from build123d import *

# Parameters (mm, degrees)
SKETCH044_R       = 1.6
PAD025_DEPTH      = 9
FILLET013_R       = 1
SKETCH075_W       = 8
SKETCH075_H       = 3
POCKET_DEPTH      = 37.001
POCKET_DEPTH_BACK = -17.001
CHAMFER_SIZE      = 0.4


with BuildPart() as part:
    # Sketch044 → Pad025 (new body)
    with BuildSketch(Plane.YZ):
        Polygon((-10, 17), (13, 17), (13, -37), (-10, -37), (-10, -30), (10, -30), (10, 10), (-10, 10), align=None)
        with Locations((-5, 14.5)):
            Circle(SKETCH044_R, mode=Mode.SUBTRACT)
        with Locations((5, 14.5)):
            Circle(SKETCH044_R, mode=Mode.SUBTRACT)
        with Locations((-5, -34.5)):
            Circle(SKETCH044_R, mode=Mode.SUBTRACT)
        with Locations((5, -34.5)):
            Circle(SKETCH044_R, mode=Mode.SUBTRACT)
    extrude(amount=-PAD025_DEPTH)

    # Fillet013
    fillet013_edges = [part.edges().sort_by_distance(p)[0] for p in [
        (-4.5, -10, 17),
        (-4.5, -10, 10),
        (-4.5, -10, -30),
        (-4.5, -10, -37),
        (-4.5, 13, -37),
        (-4.5, 13, 17),
    ]]
    fillet(fillet013_edges, radius=FILLET013_R)

    # Sketch075 (on XY_Plane042 of Origin045) → Pocket (cut, two sides)
    with BuildSketch(Plane.XY) as pocket_sk:
        Rectangle(SKETCH075_W, SKETCH075_H)
    extrude(amount=-POCKET_DEPTH, mode=Mode.SUBTRACT)
    extrude(pocket_sk.sketch, amount=-POCKET_DEPTH_BACK, mode=Mode.SUBTRACT)

    # Chamfer
    chamfer_edges = [part.edges().sort_by_distance(p)[0] for p in [
        (0, 6.75, 17),
        (0, 12.707107, 16.707107),
        (0, 13, -10),
        (0, 12.707107, -36.707107),
        (0, 6.75, -37),
        (0, 1.5, -33.5),
        (0, 5.75, -30),
        (0, 10, -10),
        (0, 5.75, 10),
        (0, 1.5, 13.5),
        (0, 3.4, -34.5),
        (0, 3.4, 14.5),
        (0, -5.25, 17),
        (0, -1.5, 13.5),
        (0, -5.25, 10),
        (0, -9.707107, 10.292893),
        (0, -10, 13.5),
        (0, -9.707107, 16.707107),
        (0, -6.6, 14.5),
        (0, -1.5, -33.5),
        (0, -5.25, -37),
        (0, -9.707107, -36.707107),
        (0, -10, -33.5),
        (0, -9.707107, -30.292893),
        (0, -5.25, -30),
        (0, -6.6, -34.5),
        (-9, 1.5, 17),
        (-9, -9.707107, 16.707107),
        (-9, 12.707107, 16.707107),
        (-9, -10, 13.5),
        (-9, 13, -10),
        (-9, -9.707107, 10.292893),
        (-9, 12.707107, -36.707107),
        (-9, 0.5, 10),
        (-9, 1.5, -37),
        (-9, 10, -10),
        (-9, -9.707107, -36.707107),
        (-9, 0.5, -30),
        (-9, -10, -33.5),
        (-9, -9.707107, -30.292893),
        (-9, -6.6, 14.5),
        (-9, 3.4, 14.5),
        (-9, -6.6, -34.5),
        (-9, 3.4, -34.5),
    ]]
    chamfer(chamfer_edges, length=CHAMFER_SIZE)


solid = part.part
Geometry: final body of the model. Coordinates: model frame, mm. A direction names the side the tool comes from. Give positions to 0.01 mm unless a question says otherwise; leave off trailing zeros. Order: outer loops, then holes, each group sorted by start corner. A loop starts at its lowest first (then second) coordinate and runs counter-clockwise, first axis right, second up. Notation, with made-up numbers: (39.25, -7) -> (81.25, -7) arc R28 ccw to (81.25, 12) -> close; hole circle Ø9 at (-39.75, 72.5). An arc over 180 degrees is marked (long way). Answer as a JSON object with one key per item and string values.
Q1. Section B-B (y = 9.5). Output: boundary loops of the cut face in (x, z), plus the area to 3 significant figures.
Entries:
{"outline": "(-9, -36.6) -> (-8.6, -37) -> (-0.4, -37) -> (0, -36.6) -> (0, -30.4) -> (-0.4, -30) -> (-8.6, -30) -> (-9, -30.4) -> close; (-9, 10.4) -> (-8.6, 10) -> (-0.4, 10) -> (0, 10.4) -> (0, 16.6) -> (-0.4, 17) -> (-8.6, 17) -> (-9, 16.6) -> close", "area": "125 mm^2"}
Q2. Material intervals for probe 1 along Z at (x, y) = (-5, 5); probe 2 along Z at (x, y) = (-1.75, -8.25); probe 3 along Y at (x, z) = (-5.5, -33.5), sorted ascending.
Entries:
{"probe 1": "z = -37 to -36.1, -32.9 to -30, 10 to 12.9, 16.1 to 17", "probe 2": "z = -37 to -30, 10 to 17", "probe 3": "y = -10 to -6.25, -3.75 to 3.75, 6.25 to 13"}
Q3. Section A-A (x = -3.5). Output: boundary loops of the cut face in (y, z).
Entries:
{"outline": "(-10, -36) arc R1 ccw to (-9, -37) -> (-1.5, -37) -> (-1.5, -30) -> (-9, -30) arc R1 ccw to (-10, -31) -> close; (-10, 11) arc R1 ccw to (-9, 10) -> (-1.5, 10) -> (-1.5, 17) -> (-9, 17) arc R1 ccw to (-10, 16) -> close; (1.5, -37) -> (12, -37) arc R1 ccw to (13, -36) -> (13, 16) arc R1 ccw to (12, 17) -> (1.5, 17) -> (1.5, 10) -> (10, 10) -> (10, -30) -> (1.5, -30) -> close; hole circle Ø3.2 at (-5, -34.5); hole circle Ø3.2 at (-5, 14.5); hole circle Ø3.2 at (5, -34.5); hole circle Ø3.2 at (5, 14.5)"}
Q4. Draft query along Y for faces 1 (the conical face through (-0.153, -9.538, 16.526)), 2 (the flat face through (-4, 0, 13)), 3 (the conical face through (-0.153, 12.538, -36.526)). Return one class per face: released by +Y, released by -Y, zero draft, split by the parting line, or undercut.
Entries:
{"face 1": "released by -Y", "face 2": "undercut", "face 3": "released by +Y"}
Q5. First-contact query: pin 1 (1.5 mm diameter, centred on y = -0.5, z = 14.5, fed in from +X); pin 2 (3.5 mm diameter, centred on y = 5, z = 14.5, fed in from -X); pin 3 (2 mm diameter, centred on x = -3, z = -22, fed in from -Y). Flat tips, straight axial feed; report the tip coordinate or a pass-through.
Entries:
{"pin 1": "stops at x = -4", "pin 2": "stops at x = -8.75", "pin 3": "stops at y = 10"}
Q6. Section C-C (z = -34.5). State how many separate pieces and enclosed holes the cut face has, plus the area to 3 significant figures.
Entries:
{"separate pieces": "3", "enclosed holes": "0", "area": "136 mm^2"}
Q7. Access query for faces 4 (the flat face through (-4, -10, -34)), 5 (the conical face through (-0.153, -9.526, 10.462)), 6 (the cylindrical face through (-4.557, -9.715, -30.301)). Directions: +Z, -Z, +X, -X, +Y, -Y. A direction counts if a zero-diameter tool reaches every point of the face in a straight line with its end or side. Return the directions, or none.
Entries:
{"face 4": "+Z, -Z, +X, -X, -Y", "face 5": "+X, -Y", "face 6": "+X, -X, -Y"}
